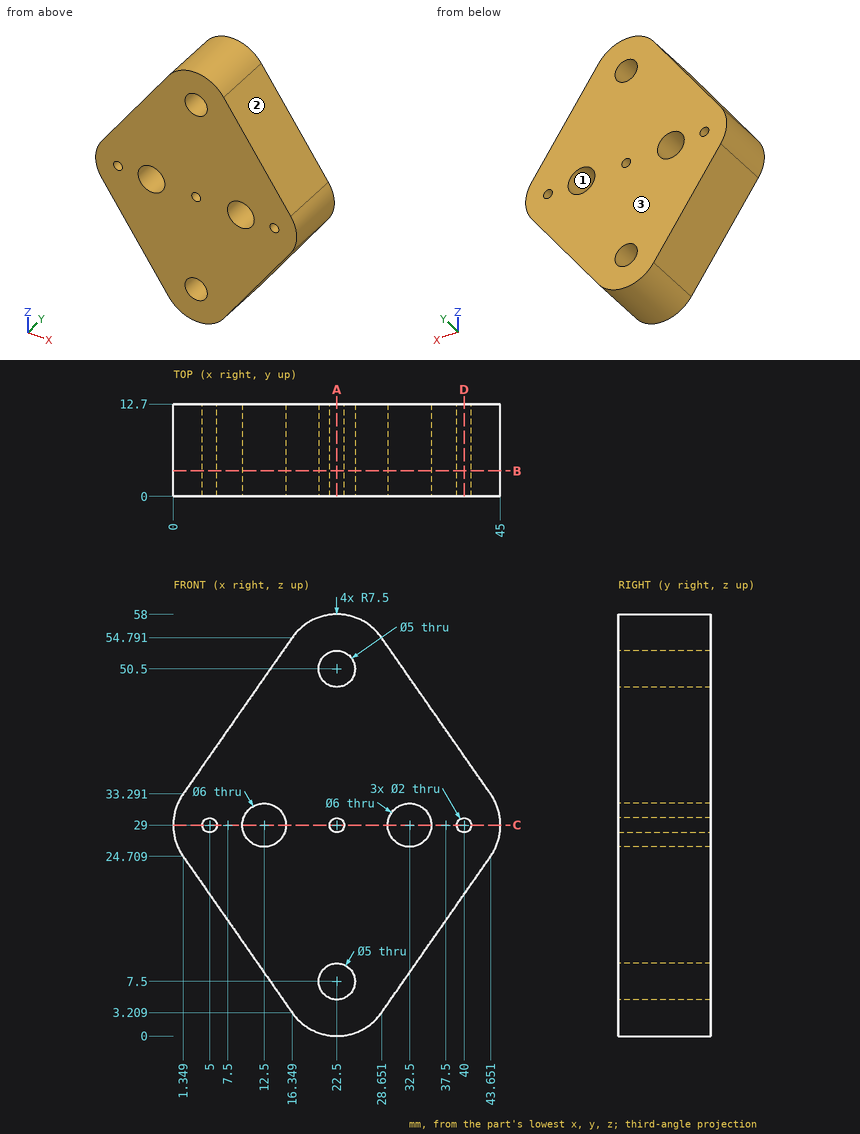
Input: dimensioned drawing with shaded views. Units: mm. Origin: part minimum x, y, z. Round coordinates to 2 decimals unless told otherwise and drop trailing zeros. Loops run counter-clockwise (first coordinate to the right, second up) from the corner with the lowest first, then second, coordinate; pieces in that order, holes last. Notation, with made-up numbers: (-14.75, 35.5) -> (31.25, 35.5) arc R24 ccw to (31.25, 57.5) -> close; hole circle Ø8 at (85, -15). An arc over 180 degrees is marked (long way). Answer as a JSON object with one key per item and string values. Group by question number.
Q1. Mould query, pull axis X, two halves, no side actions, for the marked faces 1, 2 and 3. Classes: pulls with the +X half, pulls with the -X half, needs draft (parallel to the pull), parting line crosses it, or undercut.
Q2. Section query B-B (y = 3.5). Output: boundary loops of the cut face in (x, z), plus the area to 3 significant figures.
Q3. Section query D-D (x = 40). Output: boundary loops of the cut face in (y, z) (1 decimal).
Q4. Contact query for flat-ended pins moving along their axis: P1, Ø5, axis at x = 12.5, z = 29, coming from the -Y side; P2, Ø2, axis at x = 29, y = 10.5, coming from the +Z side; P3, Ø2, axis at x = 13, y = 2, coming from the -Z side (1 decimal); P4, Ø6, axis at x = 10.5, y = 8, coming from the -Z side. Output: stop coordinate, or through.
Q5. Section query C-C (z = 29). Output: boundary loops of the cut face in (x, y), plus the area to 3 significant figures.
Q6. Section query A-A (x = 22.5). Output: boundary loops of the cut face in (y, z), plus the area to 3 significant figures.
Q7. Ray query, line 1 (X direction, y = 8.75, z = 29); line 2 (Z direction, x = 32, y = 4); line 3 (X direction, y = 8.75, z = 7.5) (1 decimal). Return the intervals inside material, ascending. Write a range as from..to.
Completed:
{
 "1": {"face 1": "undercut", "face 2": "pulls with the +X half", "face 3": "needs draft"},
 "2": {"outline": "(1.35, 24.71) -> (16.35, 3.21) arc R7.5 ccw to (28.65, 3.21) -> (43.65, 24.71) arc R7.5 ccw to (43.65, 33.29) -> (28.65, 54.79) arc R7.5 ccw to (16.35, 54.79) -> (1.35, 33.29) arc R7.5 ccw to start; hole circle Ø2 at (5, 29); hole circle Ø6 at (12.5, 29); hole circle Ø5 at (22.5, 7.5); hole circle Ø5 at (22.5, 50.5); hole circle Ø2 at (22.5, 29); hole circle Ø6 at (32.5, 29); hole circle Ø2 at (40, 29)", "area": "1,500 mm²"},
 "3": {"outline": "(0, 19.5) -> (12.7, 19.5) -> (12.7, 28) -> (0, 28) -> close; (0, 30) -> (12.7, 30) -> (12.7, 38.5) -> (0, 38.5) -> close"},
 "4": {"P1": "through", "P2": "z = 55.6", "P3": "z = 6.6", "P4": "z = 7.29"},
 "5": {"outline": "(0, 0) -> (4, 0) -> (4, 12.7) -> (0, 12.7) -> close; (6, 0) -> (9.5, 0) -> (9.5, 12.7) -> (6, 12.7) -> close; (15.5, 0) -> (21.5, 0) -> (21.5, 12.7) -> (15.5, 12.7) -> close; (23.5, 0) -> (29.5, 0) -> (29.5, 12.7) -> (23.5, 12.7) -> close; (35.5, 0) -> (39, 0) -> (39, 12.7) -> (35.5, 12.7) -> close; (41, 0) -> (45, 0) -> (45, 12.7) -> (41, 12.7) -> close", "area": "343 mm²"},
 "6": {"outline": "(0, 0) -> (12.7, 0) -> (12.7, 5) -> (0, 5) -> close; (0, 10) -> (12.7, 10) -> (12.7, 28) -> (0, 28) -> close; (0, 30) -> (12.7, 30) -> (12.7, 48) -> (0, 48) -> close; (0, 53) -> (12.7, 53) -> (12.7, 58) -> (0, 58) -> close", "area": "584 mm²"},
 "7": {"line 1": "0..4, 6..9.5, 15.5..21.5, 23.5..29.5, 35.5..39, 41..45", "line 2": "8.01..26.04, 31.96..49.99", "line 3": "13.4..20, 25..31.6"}
}
